Can you work these out from the model? Positions are in its coordinate system, mm. Face numbers are marked on the shaded views. A direction names the side the tool comes from. Give positions to 0.01 mm unless a question says otherwise; leave off trailing zeros. Order: outer loops, then holes, each group sorted by start corner. A loop starts at its lowest first (then second) coordinate and runs counter-clockwise, first axis right, second up. Notation, with made-up numbers: (12.5, 1) -> (28.5, 1) arc R13 cw to (28.5, 12) -> close; hole circle Ø4 at (69, 73.5). An arc over 180 degrees is marked (long way). Answer as a JSON object with one key per item and string values.
Autodesk Inventor part; units mm, degrees
ref_plane "YZ Plane" through (0, 0, 0) normal (1, 0, 0) x (0, 1, 0)
ref_plane "XZ Plane" through (0, 0, 0) normal (0, 1, 0) x (-1, 0, 0)
ref_plane "XY Plane" through (0, 0, 0) normal (0, 0, 1) x (1, 0, 0)
sketch "Skizze1" plane through (0, 0, 0) normal (1, 0, 0) x (0, 1, 0)
  line L0 (4, 0) -> (4, 3)
  arc A0 (4, 3) -> (3, 4) centre (3, 3) ccw
  line L1 (3, 4) -> (0, 4)
  line L2 (0, 4) -> (0, 5)
  line L3 (0, 5) -> (-3, 5)
  line L4 (-3, 5) -> (-3, 2)
  line L5 (0, 0) -> (4, 0)
  line L6 (-3, 2) -> (-3, 0)
  line L7 (-3, 0) -> (0, 0)
  point P0 (0, 2)
  dimension "d0" = 2
  dimension "d1" = 4
  dimension "d2" = 3
  dimension "d3" = 5
  dimension "d4" = 3
  dimension "d5" = 1
  dimension "d6" = 1
revolve "Umdrehung1" add sketch "Skizze1" angle 360 about axis through (0, 0, 0) along (0, 1, 0)
sketch "Skizze2" plane through (0, 4, 0) normal (0, 1, 0) x (1, 0, 0)
  line L0 (-1.9622, -1.4344) -> (-1.9622, 1.4984) construction
  line L1 (-1.9622, 1.4984) -> (1.5378, 1.4984) construction
  line L2 (1.5378, 1.4984) -> (1.5378, -1.4344) construction
  line L3 (1.5378, -1.4344) -> (-1.9622, -1.4344) construction
  line L4 (1.5378, -1.457) -> (-1.9622, -0.2771)
  line L5 (-1.9622, -0.2771) -> (-1.9622, 0.2958)
  line L6 (-1.9622, 0.2958) -> (1.5378, 1.4757)
  line L7 (1.5378, 1.4757) -> (1.5378, 0.985)
  line L8 (1.5378, 0.985) -> (0.5593, 0.6673)
  line L9 (0.5593, 0.6673) -> (0.5593, -0.6686)
  line L10 (0.5593, -0.6686) -> (1.5378, -0.9862)
  line L11 (1.5378, -0.9862) -> (1.5378, -1.457)
  line L12 (0.1622, 0.5397) -> (-1.4857, -0.002)
  line L13 (-1.4857, -0.002) -> (0.1622, -0.5409)
  line L14 (0.1622, -0.5409) -> (0.1622, 0.5397)
  point P0 (0, 0)
extrude "Extrusion1" cut sketch "Skizze2" against normal blind 0.5
sketch "Skizze4" plane through (0, -3, 0) normal (0, -1, 0) x (1, 0, 0)
  line L0 (0.75, 6.8364) -> (-0.75, 6.8364)
  line L1 (-0.75, 6.8364) -> (-0.75, 4.8364)
  line L2 (-0.75, 4.8364) -> (0.75, 4.8364)
  line L3 (0.75, 4.8364) -> (0.75, 6.8364)
  point P0 (0, 0)
  dimension "d15" = 1.5
  dimension "d16" = 2
  dimension "d19" = 0.75
extrude "Extrusion3" add sketch "Skizze4" against normal blind 3
properties part number "ButtonA_neu"
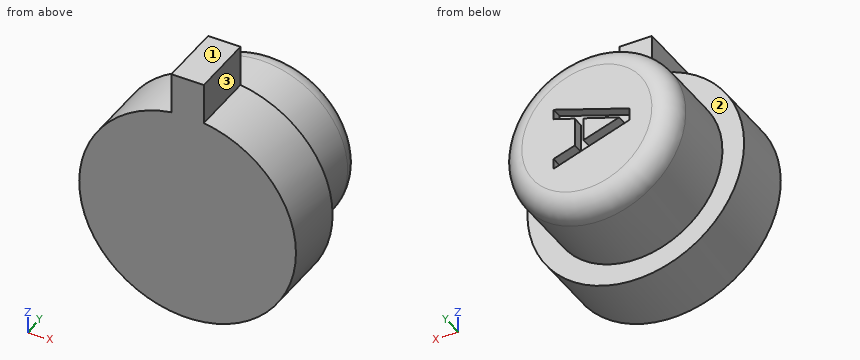
1. If we section it at A-A on y = -1.25: Please give me the cut outline in (x, z), then the cut area to 3 significant figures.
Worked answers:
{"outline": "(-0.75, 4.94) arc R5 ccw (long way) to (0.75, 4.94) -> (0.75, 6.84) -> (-0.75, 6.84) -> close", "area": "81.3 mm²"}
2. Please list where these lines run through material, in increasing order: L1, parallel to Y at x = -0.75, z = -3; L2, parallel to Y at x = -0.25, z = 4.5; L3, parallel to Z at x = 3, y = -2.
Worked answers:
{"L1": "-3 to 4", "L2": "-3 to 0", "L3": "-4 to 4"}
3. If we section it at D-D on y = 2.75: Please give me the cut outline in (x, z), then the cut area to 3 significant figures.
Worked answers:
{"outline": "circle Ø8 at (0, 0)", "area": "50.3 mm²"}
4. If we section it at C-C on z = 4.75: Please give me the cut outline in (x, y), then the cut area to 3 significant figures.
Worked answers:
{"outline": "(-1.56, -3) -> (1.56, -3) -> (1.56, 0) -> (-1.56, 0) -> close", "area": "9.37 mm²"}
5. For the marked faces 1, 2 and 3, which set-ups out of +Z, -Z, +X, -X, +Y, -Y let a thin tool reach every point of the face, with its end or its side?
Worked answers:
{"face 1": "+Z, +X, -X, +Y, -Y", "face 2": "+Y", "face 3": "+Z, +X, +Y, -Y"}
6. Will these pins go through, and if not, where does the flat tip stop? pin 1 Ø0.6 at (y, z) = (-2, 5.5) entering from +X; pin 2 Ø0.6 at (y, z) = (-2, 5.5) entering from -X; pin 3 Ø0.5 at (y, z) = (4, -1.5) entering from -X; pin 4 Ø1.5 at (x, z) = (-2.5, 5.5) entering from +Y.
Worked answers:
{"pin 1": "x = 0.75", "pin 2": "x = -0.75", "pin 3": "x = -3.36", "pin 4": "through"}
7. If we section it at B-B on x = 0: Please give me the cut outline in (y, z), then the cut area to 3 significant figures.
Worked answers:
{"outline": "(-3, -5) -> (0, -5) -> (0, -4) -> (3, -4) arc R1 ccw to (4, -3) -> (4, -0.96) -> (3.5, -0.96) -> (3.5, -0.49) -> (4, -0.49) -> (4, 0.49) -> (3.5, 0.49) -> (3.5, 0.94) -> (4, 0.94) -> (4, 3) arc R1 ccw to (3, 4) -> (0, 4) -> (0, 6.84) -> (-3, 6.84) -> close", "area": "66.6 mm²"}
